Drawing for the job (mm, zero at the part's lowest x, y, z). A direction names the side the tool comes from. Coordinates: 2 decimals unless noted, no trailing zeros. Put each result on its own line as item: value. Start each with the question number.
Q1. Drop a flat-ended pin along its axis: pin 1 (1.9 mm diameter, centred on y = 3.18, z = 1.59, fed in from +X). Give the stop position or say it passes through.
Q2. Which spindle directions (+Z, -Z, +X, -X, +Y, -Y) get a long thin tool onto all of the face, cutting with end or side? Do the marked faces 4 and 5. Say none if no direction does.
Q3. Pull direction X, two halves, no side cores. Call the marked faces 1, 2 and 3: pulls with the +X half, pulls with the -X half, needs draft (parallel to the pull), parting line crosses it, or undercut.
Q4. Drill centre lines: line 1 along X through (y, z) = (3, 5); line 2 along Z through (x, y) = (2, 3.75) (1 decimal); line 3 along Y through (x, z) = (6, 0.75). Where is each one in solid material? Low to high.
Q5. Cut at C-C (z = 5.5). Give the number of separate pieces and of enclosed holes in the cut face.
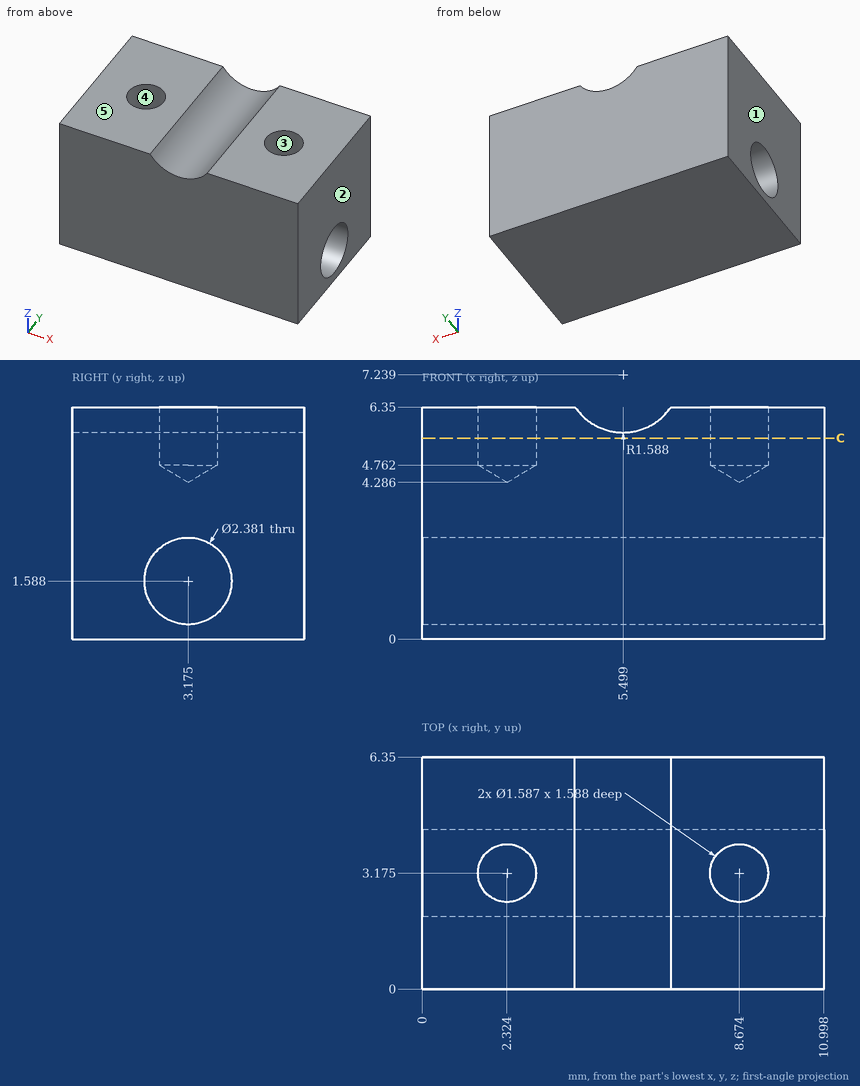
Computed values:
1. pin 1: through
2. face 4: +Z
2. face 5: +Z, +X, -X, +Y, -Y
3. face 1: pulls with the -X half
3. face 2: pulls with the +X half
3. face 3: undercut
4. line 1: 0 to 1.55, 3.1 to 7.9, 9.45 to 11
4. line 2: 0 to 0.5, 2.6 to 4.7
4. line 3: 0 to 2.33, 4.02 to 6.35
5. separate pieces: 1
5. enclosed holes: 2
